Work out the finished part from the listing and answer in its coordinate system (mm). Face numbers are marked on the shaded views. A direction names the side the tool comes from. Coordinates: 2 decimals unless noted, no trailing zeros. Order: outer loops, then holes, each group sorted by start corner. A loop starts at its lowest first (then second) coordinate and runs counter-clockwise, first axis right, second up.
```python
from build123d import *

# Parameters (mm, degrees)
CYLINDER_R     = 2
CYLINDER_DEPTH = 10
BOX_W          = 1
BOX_H          = 10
BOX_DEPTH      = 10


with BuildPart() as cilindre:
    # Cylinder → Cylinder (new body)
    with BuildSketch(Plane.XY):
        Circle(CYLINDER_R)
    extrude(amount=CYLINDER_DEPTH)


with BuildPart() as cub:
    # Box → Box (new body)
    with BuildSketch(Plane(origin=(-0.5, -4, 1.2), x_dir=(1, 0, 0), z_dir=(0, 0, 1))):
        with Locations((0.5, 5)):
            Rectangle(BOX_W, BOX_H)
    extrude(amount=BOX_DEPTH)


with BuildPart() as fusion:
    # Cone → Cone (revolve)
    with BuildSketch(Plane.XZ):
        Polygon((0, 0), (2, 0), (2.8, 2.2), (0, 2.2), align=None)
    revolve(axis=Axis((0, 0, 0), (0, 0, 1)))

    # Cut: cut Cub
    add(cub.part, mode=Mode.SUBTRACT)


with BuildPart() as fusion_1:
    # Cut placement: moved
    add(fusion.part.moved(Location((0, 0, 10))))

    # Fusion: union Cilindre
    add(cilindre.part)


solid = fusion_1.part
```
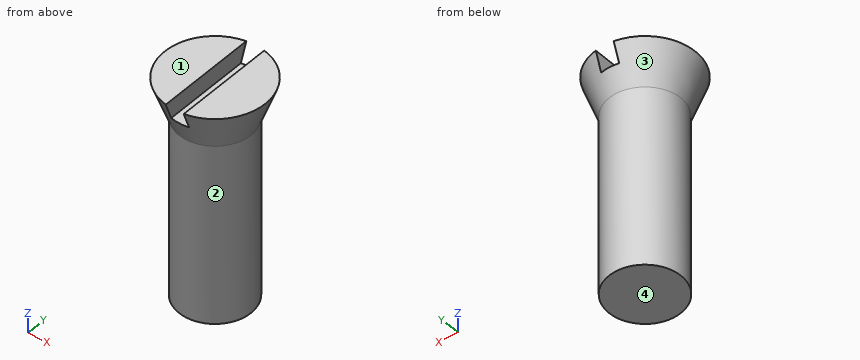
1. The part is cut by section B-B (x = 0). Determine the outline of the cut face in (y, z).
2. Consider probe 1 along X at (y, z) = (1.5, 11.5); probe 2 along X at (y, z) = (-1, 11.5); probe 3 along Z at (x, y) = (0.1, -1.5). Determine where each line is inside the solid, lowest interval first.
3. The part is cut by section C-C (z = 5.5). Determine the outline of the cut face in (x, y), plus the area to 3 significant figures.
4. The part is cut by section A-A (y = 0). Determine the outline of the cut face in (x, z).
5. The mould has two halves that part along Y. Classify the marked faces 3 and 4: released by +Y, released by -Y, zero draft, split by the parting line, or undercut.
6. Flat-ended cylindrical pins translate along their axes: pin 1 (3 mm diameter, centred on y = 2, z = 9, fed in from -X); pin 2 (0.5 mm diameter, centred on x = 0, y = 0.5, fed in from +Z); pin 3 (1 mm diameter, centred on x = 1, z = 2.5, fed in from -Y). Find the tip coordinate at first contact, or state that the pin passes through.
7. For the marked faces 1 and 2, determine the directions among +Z, -Z, +X, -X, +Y, -Y from which every point of the face is accessible in a straight line to the end or side of a thin tool.
Worked out:
1. outline: (-2.44, 11.2) - (-2, 10) - (-2, 0) - (2, 0) - (2, 10) - (2.44, 11.2) - close
2. probe 1: x = -2.06 to -0.5, 0.5 to 2.06
2. probe 2: x = -2.34 to -0.5, 0.5 to 2.34
2. probe 3: z = 0 to 11.2
3. outline: circle Ø4 at (0, 0)
3. area: 12.6 mm2
4. outline: (-2.8, 12.2) - (-2, 10) - (-2, 0) - (2, 0) - (2, 10) - (2.8, 12.2) - (0.5, 12.2) - (0.5, 11.2) - (-0.5, 11.2) - (-0.5, 12.2) - close
5. face 3: split by the parting line
5. face 4: zero draft
6. pin 1: stops at x = -1.94
6. pin 2: stops at z = 11.2
6. pin 3: stops at y = -1.94
7. face 1: +Z, +X, -X, +Y, -Y
7. face 2: -Z
